Autodesk Inventor part; units mm, degrees
ref_plane "YZ Plane" through (0, 0, 0) normal (1, 0, 0) x (0, 1, 0)
ref_plane "XZ Plane" through (0, 0, 0) normal (0, 1, 0) x (-1, 0, 0)
ref_plane "XY Plane" through (0, 0, 0) normal (0, 0, 1) x (1, 0, 0)
sketch "Sketch1" plane through (0, 0, 0) normal (0, 1, 0) x (-1, 0, 0)
  line L0 (-10.5, 12.5) -> (7.5, 12.5)
  line L1 (12.5, 7.5) -> (12.5, -7.5)
  line L2 (7.5, -12.5) -> (-10.5, -12.5)
  line L3 (-12.5, 12.5) -> (12.5, -12.5) construction
  line L4 (12.5, 12.5) -> (-12.5, -12.5) construction
  line L5 (2.5, -7.5) -> (-12.5, -7.5)
  line L6 (-12.5, 7.5) -> (2.5, 7.5)
  line L7 (2.5, 7.5) -> (2.5, -7.5)
  line L8 (2.5, -7.5) -> (-8.1051, -8.1051) construction
  line L9 (1.2546, -1.2546) -> (2.5, 7.5) construction
  line L10 (-12.5, -10.5) -> (-12.5, -7.5)
  line L11 (-12.5, 7.5) -> (-12.5, 10.5)
  arc A0 (12.5, 7.5) -> (7.5, 12.5) centre (7.5, 7.5) ccw
  arc A1 (7.5, -12.5) -> (12.5, -7.5) centre (7.5, -7.5) ccw
  arc A2 (-10.5, 12.5) -> (-12.5, 10.5) centre (-10.5, 10.5) ccw
  arc A3 (-12.5, -10.5) -> (-10.5, -12.5) centre (-10.5, -10.5) ccw
  point P0 (0, 0)
  point P1 (-12.5, -9)
  dimension "d0" = 5
  dimension "d1" = 2
  dimension "d2" = 15
  dimension "d3" = 25
  dimension "d7" = 15
  dimension "d8" = 25
extrude "Extrusion1" add sketch "Sketch1" along normal blind 8
sketch "Sketch2" plane through (-7.5, 0, 12.5) normal (0, 0, 1) x (1, 0, 0)
  circle A0 centre (15, 4) radius 2.75
  line L0 (0, 8) -> (18, 8)
  line L1 (18, 0) -> (18, 8)
  point P0 (7.5, 0)
  dimension "d9" = 5.5
  dimension "d10" = 4
  dimension "d26" = 3
extrude "Extrusion2" cut sketch "Sketch2" against normal blind 44.5
sketch "Sketch4" plane through (0, 0, 0) normal (0, -1, 0) x (1, 0, 0)
  line L0 (-13.6886, 6.5298) -> (-6.3114, 6.5298)
  line L1 (-6.3114, 6.5298) -> (-6.3114, -6.5298)
  line L2 (-6.3114, -6.5298) -> (-13.6886, -6.5298)
  line L3 (-18.6886, -1.5298) -> (-18.6886, 1.5298)
  line L4 (-12.5, -7.5) -> (-12.5, 7.5)
  line L5 (-18.6886, 6.5298) -> (-6.3114, -6.5298) construction
  line L6 (-6.3114, 6.5298) -> (-18.6886, -6.5298) construction
  arc A0 (-18.6886, -1.5298) -> (-13.6886, -6.5298) centre (-13.6886, -1.5298) ccw
  arc A1 (-13.6886, 6.5298) -> (-18.6886, 1.5298) centre (-13.6886, 1.5298) ccw
  point P0 (0, 0)
  point P1 (-12.5, 0)
  dimension "d13" = 5
extrude "Extrusion3" add sketch "Sketch4" against normal blind 8
sketch "Sketch5" plane through (0, 0, 0) normal (0, -1, 0) x (1, 0, 0)
  line L0 (-10.0746, -4.0008) -> (-14.6934, -4.0008)
  line L1 (-14.6934, -4.0008) -> (-17.0028, -0.0008)
  line L2 (-17.0028, -0.0008) -> (-14.6934, 3.9992)
  line L3 (-14.6934, 3.9992) -> (-10.0746, 3.9992)
  line L4 (-10.0746, 3.9992) -> (-7.7652, -0.0008)
  line L5 (-7.7652, -0.0008) -> (-10.0746, -4.0008)
  line L6 (-7.5, 12.5) -> (10.5, 12.5)
  circle A0 centre (-12.384, -0.0008) radius 2.75
  point P0 (0, 0)
  dimension "d16" = 8
  dimension "d17" = 5.5
extrude "Extrusion4" cut sketch "Sketch5" against normal blind 8 contours A0
sketch "Sketch7" plane through (0, 0, 0) normal (0, -1, 0) x (1, 0, 0)
  circle A0 centre (-12.384, -0.0008) radius 2.75
  line L0 (-7.7652, -0.0008) -> (-10.0746, -4.0008)
  line L1 (-10.0746, -4.0008) -> (-14.6934, -4.0008)
  line L2 (-14.6934, -4.0008) -> (-17.0028, -0.0008)
  line L3 (-17.0028, -0.0008) -> (-14.6934, 3.9992)
  line L4 (-14.6934, 3.9992) -> (-10.0746, 3.9992)
  line L5 (-10.0746, 3.9992) -> (-7.7652, -0.0008)
  line L6 (-7.5, 12.5) -> (10.5, 12.5)
  point P0 (0, 0)
  point P1 (-12.384, 3.9992)
  dimension "d22" = 8
extrude "Extrusion5" cut sketch "Sketch7" against normal blind 2 contours A0 | L0 L1 L2 L3 L4 L5
ref_plane "Work Plane1" through (0, 4, 0) normal (0, -1, 0) x (1, 0, 0)
mirror "Mirror1" about plane through (0, 4, 0) normal (0, -1, 0) of "Extrusion5"
properties part number "J1"
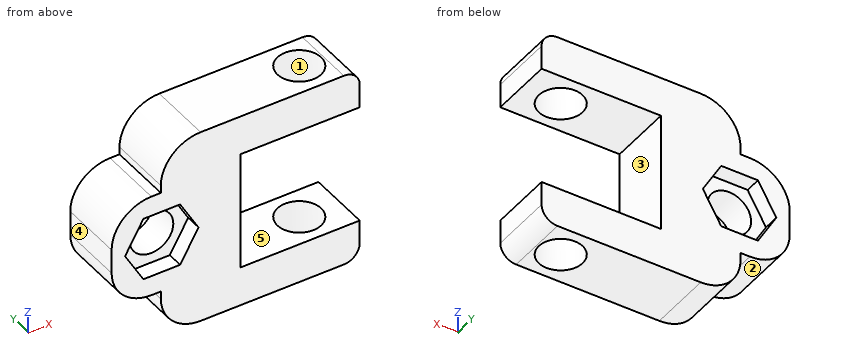
Design review of the part built by this model. Coordinates are the model's own, in mm. Face numbers are marked on the shaded views. A direction names the side the tool comes from. Coordinates: 2 decimals unless noted, no trailing zeros. Loops run counter-clockwise (first coordinate to the right, second up) from the corner with the lowest first, then second, coordinate; pieces in that order, holes last.
Q1. We need section B-B on x = 7.5. State the section outline as (y, z) points.
Reported:
outline: (0, -12.5) - (1.25, -12.5) - (1.25, -7.5) - (0, -7.5) - close; (0, 7.5) - (1.25, 7.5) - (1.25, 12.5) - (0, 12.5) - close; (6.75, -12.5) - (8, -12.5) - (8, -7.5) - (6.75, -7.5) - close; (6.75, 7.5) - (8, 7.5) - (8, 12.5) - (6.75, 12.5) - close
Q2. For pin 1 (2 mm diameter, centred on x = -14.5, y = 2.5, fed in from +Z); pin 2 (2 mm diameter, centred on x = -12, y = 7, fed in from +Z); pin 3 (0.5 mm diameter, centred on y = 3.5, z = 7, fed in from -X), all flat-tipped, find the tip position at first contact; note any pin that passes through.
Reported:
pin 1: stops at z = 6.53
pin 2: stops at z = 11.07
pin 3: stops at x = -12.5
Q3. We need section A-A on y = 4. State the section outline as (x, z) points.
Reported:
outline: (-18.69, -1.53) arc R5 ccw to (-13.69, -6.53) - (-12.5, -6.53) - (-12.5, -7.5) arc R5 ccw to (-7.5, -12.5) - (4.75, -12.5) - (4.75, -7.5) - (-2.5, -7.5) - (-2.5, 7.5) - (4.75, 7.5) - (4.75, 12.5) - (-7.5, 12.5) arc R5 ccw to (-12.5, 7.5) - (-12.5, 6.53) - (-13.69, 6.53) arc R5 ccw to (-18.69, 1.53) - close; (10.25, -12.5) - (10.5, -12.5) arc R2 ccw to (12.5, -10.5) - (12.5, -7.5) - (10.25, -7.5) - close; (10.25, 7.5) - (12.5, 7.5) - (12.5, 10.5) arc R2 ccw to (10.5, 12.5) - (10.25, 12.5) - close; hole circle Ø5.5 at (-12.38, 0)
Q4. We need section C-C on x = 0.5. State the section outline as (y, z) points, and give its area (3 significant figures).
Reported:
outline: (0, -12.5) - (8, -12.5) - (8, -7.5) - (0, -7.5) - close; (0, 7.5) - (8, 7.5) - (8, 12.5) - (0, 12.5) - close
area: 80.0 mm2
Q5. The part is to be moulded in two halves that separate along Z. For the marked faces 1, 2 and 3, say which applies: +Z half, -Z half, draft (parallel to the pull), parting line (faces both ways), or undercut.
Reported:
face 1: draft
face 2: -Z half
face 3: undercut
Q6. Tool access review of the marked faces 4 and 5: name each direction out of +Z, -Z, +X, -X, +Y, -Y from which nothing blocks a thin tool from reaching the whole face with its end or side.
Reported:
face 4: +Z, -Z, -X, +Y, -Y
face 5: +X, +Y, -Y
Q7. To check wall thickness, follow line 1 (Z direction, x = 3, y = 5); line 2 (Y direction, x = 7.5, z = -9.45); line 3 (Z direction, x = -9.5, y = 0.75). State the ranges of each line that lie inside material, in increasing order.
Reported:
line 1: z = -12.5 to -7.5, 7.5 to 12.5
line 2: y = 0 to 1.25, 6.75 to 8
line 3: z = -12.08 to -3.01, 3 to 12.08
Q8. We need section D-D on z = 0.5. State the section outline as (x, y) points.
Reported:
outline: (-18.69, 0) - (-16.71, 0) - (-16.71, 2) - (-15.09, 2) - (-15.09, 6) - (-16.71, 6) - (-16.71, 8) - (-18.69, 8) - close; (-9.68, 2) - (-8.05, 2) - (-8.05, 0) - (-2.5, 0) - (-2.5, 8) - (-8.05, 8) - (-8.05, 6) - (-9.68, 6) - close
